```python
from build123d import *

# Parameters (mm, degrees)
F0_R     = 3.175
F0_W     = 38.1
F0_H     = 38.1
F1_DEPTH = 6.35
F2_R     = 25.4
F3_R     = 5.08
F4_R     = 7.62
F5_R     = 5.08


with BuildPart() as f1:
    # F0 (on Top) → F1 (new body)
    with BuildSketch(Plane.XY):
        Polygon((149.225, -25.4), (-149.225, -25.4), (-149.225, -35.56), (-149.225, -138.1431958742), (-71.8420489686, -215.5261469057), (71.8420489686, -215.5261469057), (149.225, -138.1431958742), (149.225, -31.75), align=None)
        with Locations((-101.55326548, -167.8544181521)):
            Circle(F0_R, mode=Mode.SUBTRACT)
        with Locations((-50.799996416, -157.1931958742)):
            Circle(F0_R, mode=Mode.SUBTRACT)
        with Locations((-130.175, -125.4431958742)):
            Circle(F0_R, mode=Mode.SUBTRACT)
        with Locations((0, -125.4431958742)):
            Rectangle(F0_W, F0_H, mode=Mode.SUBTRACT)
        with Locations((-50.799996416, -93.6931958742)):
            Circle(F0_R, mode=Mode.SUBTRACT)
        with Locations((-50.165, -63.5)):
            Circle(F0_R, mode=Mode.SUBTRACT)
        with Locations((50.799996416, -157.1931958742)):
            Circle(F0_R, mode=Mode.SUBTRACT)
        with Locations((101.5532683632, -167.8544152689)):
            Circle(F0_R, mode=Mode.SUBTRACT)
        with Locations((50.799996416, -93.6931958742)):
            Circle(F0_R, mode=Mode.SUBTRACT)
        with Locations((130.175, -125.4431958742)):
            Circle(F0_R, mode=Mode.SUBTRACT)
        with Locations((50.165, -63.5)):
            Circle(F0_R, mode=Mode.SUBTRACT)
        Polygon((-149.225, 35.56), (-149.225, 25.4), (149.225, 25.4), (149.225, 31.75), (149.225, 138.1431958742), (110.5335244843, 176.8346713899), (71.8420489686, 215.5261469057), (-71.8420489686, 215.5261469057), (-110.5335216011, 176.8346742731), (-149.225, 138.1431958742), align=None)
        with Locations((-50.165, 63.5)):
            Circle(F0_R, mode=Mode.SUBTRACT)
        with Locations((-130.175, 125.4431958742)):
            Circle(F0_R, mode=Mode.SUBTRACT)
        with Locations((-50.799996416, 93.6931958742)):
            Circle(F0_R, mode=Mode.SUBTRACT)
        Polygon((0, 106.3931958742), (-19.05, 106.3931958742), (-19.05, 144.4931958742), (19.05, 144.4931958742), (19.05, 106.3931958742), align=None, mode=Mode.SUBTRACT)
        with BuildLine():
            ThreePointArc((-98.37826548, 167.8544181521), (-102.7682853778, 164.9211006363), (-103.7983295103, 170.0994821823))
            ThreePointArc((-103.7983295103, 170.0994821823), (-100.3382455823, 170.7877356678), (-98.37826548, 167.8544181521))
        make_face(mode=Mode.SUBTRACT)
        with Locations((-50.799996416, 157.1931958742)):
            Circle(F0_R, mode=Mode.SUBTRACT)
        with Locations((50.165, 63.5)):
            Circle(F0_R, mode=Mode.SUBTRACT)
        with Locations((50.799996416, 93.6931958742)):
            Circle(F0_R, mode=Mode.SUBTRACT)
        with Locations((130.175, 125.4431958742)):
            Circle(F0_R, mode=Mode.SUBTRACT)
        with Locations((50.799996416, 157.1931958742)):
            Circle(F0_R, mode=Mode.SUBTRACT)
        with BuildLine():
            ThreePointArc((104.7282683632, 167.8544152689), (98.6199508475, 166.6393953711), (103.7983323935, 170.0994792991))
            ThreePointArc((103.7983323935, 170.0994792991), (104.4865858789, 169.0694351666), (104.7282683632, 167.8544152689))
        make_face(mode=Mode.SUBTRACT)
        Polygon((-149.225, -35.56), (-149.225, -25.4), (-149.225, 25.4), (-149.225, 35.56), (-159.385, 35.56), (-159.385, -35.56), align=None)
        with BuildLine():
            ThreePointArc((149.225, 25.4), (174.625, 0), (149.225, -25.4))
            Line((149.225, -25.4), (149.225, -31.75))
            ThreePointArc((149.225, -31.75), (180.975, 0), (149.225, 31.75))
            Line((149.225, 31.75), (149.225, 25.4))
        make_face()
        with Locations((-130.175, -125.4431958742)):
            Circle(F0_R)
        with Locations((-101.55326548, -167.8544181521)):
            Circle(F0_R)
        with Locations((-50.165, -63.5)):
            Circle(F0_R)
        with Locations((-50.799996416, -93.6931958742)):
            Circle(F0_R)
        with Locations((-50.799996416, -157.1931958742)):
            Circle(F0_R)
        with Locations((50.165, -63.5)):
            Circle(F0_R)
        with Locations((50.799996416, -93.6931958742)):
            Circle(F0_R)
        with Locations((50.799996416, -157.1931958742)):
            Circle(F0_R)
        with Locations((101.5532683632, -167.8544152689)):
            Circle(F0_R)
        with Locations((130.175, -125.4431958742)):
            Circle(F0_R)
        with Locations((-130.175, 125.4431958742)):
            Circle(F0_R)
        with Locations((-50.799996416, 93.6931958742)):
            Circle(F0_R)
        with Locations((-50.165, 63.5)):
            Circle(F0_R)
        with Locations((50.165, 63.5)):
            Circle(F0_R)
        with Locations((50.799996416, 93.6931958742)):
            Circle(F0_R)
        with Locations((50.799996416, 157.1931958742)):
            Circle(F0_R)
        with Locations((-50.799996416, 157.1931958742)):
            Circle(F0_R)
        with BuildLine():
            ThreePointArc((-98.37826548, 167.8544181521), (-100.3382455823, 170.7877356678), (-103.7983295103, 170.0994821823))
            ThreePointArc((-103.7983295103, 170.0994821823), (-102.7682853778, 164.9211006363), (-98.37826548, 167.8544181521))
        make_face()
        with BuildLine():
            ThreePointArc((104.7282683632, 167.8544152689), (104.4865858789, 169.0694351666), (103.7983323935, 170.0994792991))
            ThreePointArc((103.7983323935, 170.0994792991), (98.6199508475, 166.6393953711), (104.7282683632, 167.8544152689))
        make_face()
        with Locations((130.175, 125.4431958742)):
            Circle(F0_R)
    extrude(amount=F1_DEPTH)

    # F2
    f2_edges = [f1.edges().sort_by_distance(p)[0] for p in [
        (149.225, -138.143196, 3.175),
        (-149.225, -138.143196, 3.175),
        (149.225, 138.143196, 3.175),
        (-149.225, 138.143196, 3.175),
    ]]
    fillet(f2_edges, radius=F2_R)

    # F3
    f3_edges = [f1.edges().sort_by_distance(p)[0] for p in [
        (149.225, -31.75, 3.175),
        (149.225, 31.75, 3.175),
    ]]
    fillet(f3_edges, radius=F3_R)

    # F4
    f4_edges = [f1.edges().sort_by_distance(p)[0] for p in [
        (-159.385, -35.56, 3.175),
        (-159.385, 35.56, 3.175),
    ]]
    fillet(f4_edges, radius=F4_R)

    # F5
    f5_edges = [f1.edges().sort_by_distance(p)[0] for p in [
        (-149.225, -35.56, 3.175),
        (-149.225, 35.56, 3.175),
    ]]
    fillet(f5_edges, radius=F5_R)


solid = f1.part
```
Could you check a few things on this model? Use its own coordinates, in mm. Round coordinates to 2 decimals unless told otherwise and drop trailing zeros. Loops run counter-clockwise (first coordinate to the right, second up) from the corner with the lowest first, then second, coordinate; pieces in that order, holes last. Notation, with made-up numbers: M 79,64 L 112,64 A28 ccw 112,91 Z; hole C 32.25,53 d10. An arc over 180 degrees is marked long. Put each result on its own line as item: value.
Q1. Imagine slicing it at D-D (y = 48). Write out the boundary of the cut face in (x, z) (3 decimals), then the cut area to 3 significant figures.
Check result:
outline: M -149.225,0 L 149.225,0 L 149.225,6.35 L -149.225,6.35 Z
area: 1,900 mm2
Q2. Imagine slicing it at C-C (z = 3). State how many separate pieces and enclosed holes the cut face has, then the cut area to 3 significant figures.
Check result:
separate pieces: 1
enclosed holes: 3
area: 99,800 mm2
Q3. Thinking about a two-plate mould opening in Y: for faces 1 (the face through (8, 51, 0)), 2 (the face through (-107.303, -180.065, 3.131)), 3 (the face through (180.97, -0.64, 3.13)), 4 (the face through (174.62, 0.56, 3.13)), which applies, released by +Y, released by -Y, zero draft, split by the parting line, or undercut?
Check result:
face 1: zero draft
face 2: released by -Y
face 3: split by the parting line
face 4: undercut
Q4. Imagine slicing it at A-A (x = -45.5). Write out the boundary of the cut face in (y, z), then the cut area to 3 significant figures.
Check result:
outline: M -215.53,0 L -25.4,0 L -25.4,6.35 L -215.53,6.35 Z; M 25.4,0 L 215.53,0 L 215.53,6.35 L 25.4,6.35 Z
area: 2,410 mm2
Q5. Imagine slicing it at B-B (y = 0). Write out the boundary of the cut face in (x, z) (3 decimals).
Check result:
outline: M -159.385,0 L -149.225,0 L -149.225,6.35 L -159.385,6.35 Z; M 174.625,0 L 180.975,0 L 180.975,6.35 L 174.625,6.35 Z
Q6. I need wall thicknesses on probe 1 along Y at (x, z) = (-11, 0.75); probe 2 along Y at (x, z) = (43.5, 0.5); probe 3 along Y at (x, z) = (122.5, 2). Which ranges of each line are inside material? Lowest first, please.
Check result:
probe 1: -215.53 to -144.49, -106.39 to -25.4, 25.4 to 106.39, 144.49 to 215.53
probe 2: -215.53 to -25.4, 25.4 to 215.53
probe 3: -164.87 to -25.4, 25.4 to 164.87
Q7. For pin 1 (1.9 mm diameter, centred on y = -121, z = 3, fed in from -X) (3 decimals); pin 2 (3 mm diameter, centred on x = -89.5, z = 1, fed in from -Y); pin 3 (1.9 mm diameter, centred on y = 11, z = 3, fed in from +X), each with a flat end and sliding along its axis, tell me the tip position at first contact or that it passes through.
Check result:
pin 1: x = -149.225
pin 2: y = -199.37
pin 3: x = 179.34
